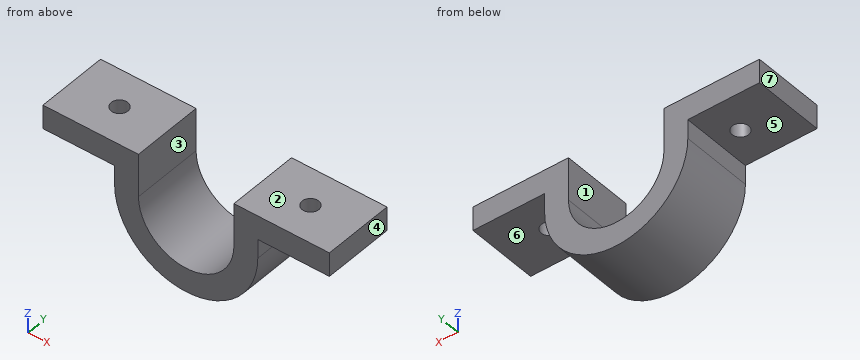
from build123d import *

# Parameters (mm, degrees)
BOSS_EXTRUDE1_DEPTH = 15
SKETCH2_R           = 1.75
CUT_EXTRUDE1_DEPTH  = 6


with BuildPart() as part:
    # Sketch1 → Boss-Extrude1 (new body)
    with BuildSketch(Plane(origin=(0, 0, 0), x_dir=(1, 0, 0), z_dir=(0, 1, 0))):
        with BuildLine():
            Line((-30, -4), (-30, -9))
            Line((-30, -9), (-10, -9))
            Line((-10, -9), (-10, 0))
            ThreePointArc((-10, 0), (0, 10), (10, 0))
            Line((10, 0), (10, -9))
            Line((10, -9), (30, -9))
            Line((30, -9), (30, -4))
            Line((30, -4), (15, -4))
            Line((15, -4), (15, 0))
            ThreePointArc((15, 0), (0, 15), (-15, 0))
            Line((-15, 0), (-15, -4))
            Line((-15, -4), (-30, -4))
        make_face()
    extrude(amount=BOSS_EXTRUDE1_DEPTH)

    # Sketch2 → Cut-Extrude1 (cut, through all)
    with BuildSketch(Plane(origin=(0, 0, 4), x_dir=(-1, 0, 0), z_dir=(0, 0, -1))):
        with Locations((-20, 7.5)):
            Circle(SKETCH2_R)
        with Locations((20, 7.5)):
            Circle(SKETCH2_R)
    extrude(amount=-CUT_EXTRUDE1_DEPTH, mode=Mode.SUBTRACT)


solid = part.part
Read the model definition and answer for the solid it produces. Units are mm, in the model's axes. Face numbers are marked on the shaded views. A direction names the side the tool comes from. Give positions to 0.01 mm unless a question says otherwise; leave off trailing zeros. Write each loop counter-clockwise with the first axis right and the second up, starting at its lowest first coordinate (ties: lowest second). Pieces come first, ordered by that corner, then holes. Notation, with made-up numbers: (12.25, -23.5) -> (45.25, -23.5) arc R25 ccw to (45.25, 13.5) -> close; hole circle Ø3 at (21, 16). An arc over 180 degrees is marked (long way). Answer as a JSON object with one key per item and string values. Group by question number.
1) A tool of negligible diameter and unlimited length cuts with its end or side. For the marked faces 5, 6 and 7, from which of +Z, -Z, +X, -X, +Y, -Y can it reach the whole face along a straight path? Write none if from no direction.
2) Each of these flat-tipped pins is pushed along its axis until it touches: P1, Ø2.5, axis at y = 9, z = 2.5, coming from the -X side; P2, Ø3, axis at x = 20, y = 7.5, coming from the +Z side; P3, Ø2, axis at x = -7.5, z = -9, coming from the -Y side; P4, Ø1, axis at y = 13.5, z = -5, coming from the -X side. Where does it stop, or does it pass through?
3) The mould has two halves that part along X. Classify the marked faces 1, 2, 3 and 4: +X half, -X half, draft (parallel to the pull), parting line (faces both ways), or undercut.
4) Find section D-D (y = 3.75). Write down the section's boundary in (x, z).
5) Consider L1, parallel to Y at x = -20, z = 7.05; L2, parallel to X at y = 7, z = 1.5; L3, parallel to X at y = 5.25, z = -3.5. Determine where each line is inside the solid, lowest interval first. Write a range as from..to.
6) Find section B-B (x = 20). Write down the section's boundary in (y, z).
7) Find section C-C (y = 7.5). Write down the section's boundary in (x, z), and give its area (3 significant figures).
8) Find section A-A (z = 2). Write down the section's boundary in (x, y), and give its area (3 significant figures).
Values follow:
{
 "1": {"face 5": "-Z, -X, +Y, -Y", "face 6": "-Z, +X, +Y, -Y", "face 7": "+Z, -Z, -X, +Y, -Y"},
 "2": {"P1": "stops at x = -15", "P2": "passes through", "P3": "stops at y = 0", "P4": "stops at x = -14.31"},
 "3": {"face 1": "undercut", "face 2": "draft", "face 3": "undercut", "face 4": "+X half"},
 "4": {"outline": "(-30, 4) -> (-15, 4) -> (-15, 0) arc R15 ccw to (15, 0) -> (15, 4) -> (30, 4) -> (30, 9) -> (10, 9) -> (10, 0) arc R10 cw to (-10, 0) -> (-10, 9) -> (-30, 9) -> close"},
 "5": {"L1": "y = 0..5.75, 9.25..15", "L2": "x = -15..-10, 10..15", "L3": "x = -14.59..-9.37, 9.37..14.59"},
 "6": {"outline": "(0, 4) -> (5.75, 4) -> (5.75, 9) -> (0, 9) -> close; (9.25, 4) -> (15, 4) -> (15, 9) -> (9.25, 9) -> close"},
 "7": {"outline": "(-30, 4) -> (-21.75, 4) -> (-21.75, 9) -> (-30, 9) -> close; (-18.25, 4) -> (-15, 4) -> (-15, 0) arc R15 ccw to (15, 0) -> (15, 4) -> (18.25, 4) -> (18.25, 9) -> (10, 9) -> (10, 0) arc R10 cw to (-10, 0) -> (-10, 9) -> (-18.25, 9) -> close; (21.75, 4) -> (30, 4) -> (30, 9) -> (21.75, 9) -> close", "area": "401 mm2"},
 "8": {"outline": "(-15, 0) -> (-10, 0) -> (-10, 15) -> (-15, 15) -> close; (10, 0) -> (15, 0) -> (15, 15) -> (10, 15) -> close", "area": "150 mm2"}
}
